```python
from build123d import *

# Parameters (mm, degrees)
SKETCH1_R           = 4.7625
BOSS_EXTRUDE1_DEPTH = 304.8
SKETCH2_W           = 12.7
SKETCH2_H           = 1.5875
CUT_EXTRUDE1_DEPTH  = 76.2


with BuildPart() as part:
    # Sketch1 → Boss-Extrude1 (new body)
    with BuildSketch(Plane(origin=(0, 0, 0), x_dir=(0, 0, -1), z_dir=(1, 0, 0))):
        Circle(SKETCH1_R)
    extrude(amount=BOSS_EXTRUDE1_DEPTH)

    # Sketch2 → Cut-Extrude1 (cut)
    with BuildSketch(Plane.ZY):
        Rectangle(SKETCH2_W, SKETCH2_H)
    extrude(amount=-CUT_EXTRUDE1_DEPTH, mode=Mode.SUBTRACT)


solid = part.part
```
Geometry check sheet. Reference: the model listing, model coordinates, mm. Give positions to 0.01 mm unless a question says otherwise; leave off trailing zeros. Order: outer loops, then holes, each group sorted by start corner. A loop starts at its lowest first (then second) coordinate and runs counter-clockwise, first axis right, second up.
1. Gauge pin test, flat ends, axial feed: pin 1 Ø2 at (x, y) = (170, 3) entering from +Z; pin 2 Ø3 at (x, y) = (201, 2) entering from +Z; pin 3 Ø3 at (x, z) = (29.5, -2.5) entering from +Y. Record the tip position at first contact, or that the pin passes through.
2. Thickness scan on L1, parallel to X at y = 0.25, z = 1; L2, parallel to Y at x = 275, z = 0.75; L3, parallel to Y at x = 67.5, z = -0.25. Record the ranges inside material, lowest first.
3. Section check B-B, the plane x = 34. Enter the section's corners in (y, z) (1 decimal), and give its area (3 significant figures).
4. Release check for a two-part mould opening along Y. For faces 1 (the face through (150.266, 1.431, -4.543)), 2 (the face through (304.8, 0, 0)), 3 (the face through (38, 0.794, 0)) record: pulls with the +Y half, pulls with the -Y half, needs draft (parallel to the pull), parting line crosses it, or undercut.
5. Section check D-D, the plane y = 3.25. Enter the section's corners in (x, z).
6. Section check A-A, the plane z = 0. Enter the section's corners in (x, y).
7. Section check C-C, the plane x = 172.5. Enter the section's corners in (y, z) (1 decimal), and give its area (3 significant figures).
Values follow:
1. pin 1: stops at z = 4.32
1. pin 2: stops at z = 4.74
1. pin 3: stops at y = 4.66
2. L1: x = 76.2 to 304.8
2. L2: y = -4.7 to 4.7
2. L3: y = -4.76 to -0.79, 0.79 to 4.76
3. outline: (-0.8, -4.7) - (-0.8, 4.7) arc R4.8 ccw to start; (0.8, -4.7) arc R4.8 ccw to (0.8, 4.7) - close
3. area: 56.2 mm2
4. face 1: parting line crosses it
4. face 2: needs draft
4. face 3: undercut
5. outline: (0, -3.48) - (304.8, -3.48) - (304.8, 3.48) - (0, 3.48) - close
6. outline: (0, -4.76) - (304.8, -4.76) - (304.8, 4.76) - (0, 4.76) - (0, 0.79) - (76.2, 0.79) - (76.2, -0.79) - (0, -0.79) - close
7. outline: circle Ø9.5 at (0, 0)
7. area: 71.3 mm2
